Read the model definition and answer for the solid it produces. Units are mm, in the model's axes. Face numbers are marked on the shaded views. A direction names the side the tool comes from. Give positions to 0.01 mm unless a question says otherwise; leave off trailing zeros. Order: outer loops, then holes, each group sorted by start corner. A loop starts at its lowest first (then second) coordinate and runs counter-clockwise, first axis right, second up.
Item 1: A cutting plane is placed at D-D (z = 7). Write down the section's boundary in (x, y), plus the area to 3 significant figures.
Item 2: Find the intervals of material crossed by line 1 along X through (y, z) = (11, 24.5); line 2 along Z through (x, y) = (32.5, 3.5); line 3 along Y through (x, z) = (24, 1), in increasing order.
Item 3: Which of the six approach directions +Z, -Z, +X, -X, +Y, -Y give full straight-line access (tool end or side, diameter ignored) to the marked faces 1, 2 and 3?
Item 4: A cutting plane is placed at C-C (y = 10). Write down the section's boundary in (x, z).
Item 5: A cutting plane is placed at B-B (x = 19.5). Write down the section's boundary in (y, z).
Item 6: Given pin 1 Ø6 at (x, z) = (34.5, 20.5) entering from +Y; pin 2 Ø1 at (x, y) = (27, 40.5) entering from -Z; pin 3 Ø6 at (x, z) = (21, 26.5) entering from +Y; pin 4 Ø2 at (y, z) = (36.5, 33.5) entering from -X, each flat-ended and moving along its own axis, determine where each tip first touches the part or whether it passes through.
Item 7: The mould has two halves that part along Y. Classify the marked faces 4, 5, 6 and 7: +Y half, -Y half, draft (parallel to the pull), parting line (faces both ways), or undercut.
Item 8: A cutting plane is placed at A-A (z = 39.5). Write down the section's boundary in (x, y), plus the area to 3 significant figures.
from build123d import *

# Parameters (mm, degrees)
BOSS_EXTRUDE1_DEPTH      = 24.000000335
SKETCH2_W                = 24.000000671
SKETCH2_H                = 21.641136132
BOSS_EXTRUDE2_DEPTH      = 14.161821686
BOSS_EXTRUDE3_DEPTH      = 2.999999665
BOSS_EXTRUDE4_DEPTH      = 21.358863868
SKETCH5_W                = 27.000000671
SKETCH5_H                = 43
BOSS_EXTRUDE5_DEPTH      = 24.000001
CUT_EXTRUDE1_DEPTH       = 6.152247735
SKETCH7_W                = 24.000000671
SKETCH7_H                = 40
CUT_EXTRUDE2_DEPTH       = 8.00957395
BOSS_EXTRUDE6_START      = 3
BOSS_EXTRUDE6_DEPTH      = 3
SKETCH9_W                = 41
SKETCH9_H                = 22.000001
CUT_EXTRUDE3_DEPTH       = 66.345237915
SKETCH10_W               = 29.947000182
SKETCH10_H               = 17
BOSS_EXTRUDE7_DEPTH      = 2
F_5_0_5_DIAMETER_HOLE1_D = 5
FILLET1_R                = 1.5
FILLET2_R                = 5
SKETCH15_R               = 1.225
BOSS_EXTRUDE8_DEPTH      = 2


with BuildPart() as part:
    # Sketch1 → Boss-Extrude1 (new body)
    with BuildSketch(Plane(origin=(18, 0, 0), x_dir=(0, -1, 0), z_dir=(-1, 0, 0))):
        with BuildLine():
            Line((-0.838178314, 3), (-0.838178314, 0))
            Line((-0.838178314, 0), (0, 0))
            ThreePointArc((0, 0), (-0.41433113, 1.501329358), (-0.838178314, 3))
        make_face()
    extrude(amount=-BOSS_EXTRUDE1_DEPTH)

    # Sketch2 → Boss-Extrude2 (add)
    with BuildSketch(Plane(origin=(0, 0.838178314, 0), x_dir=(-1, 0, 0), z_dir=(0, 1, 0))):
        with Locations((-30.000000336, 10.820568066)):
            Rectangle(SKETCH2_W, SKETCH2_H)
    extrude(amount=BOSS_EXTRUDE2_DEPTH)


with BuildPart() as boss_extrude3_tool:
    # Sketch3 → Boss-Extrude3 (new body)
    with BuildSketch(Plane(origin=(42.000000335, 0, 0), x_dir=(0, 0, -1), z_dir=(1, 0, 0))):
        with BuildLine():
            Line((0, 15), (0, 0))
            ThreePointArc((0, 0), (-10.901557165, 3.244484944), (-21.641136132, 6.99042605))
            Line((-21.641136132, 6.99042605), (-43, 15))
            Line((-43, 15), (0, 15))
        make_face()
    extrude(amount=BOSS_EXTRUDE3_DEPTH)


with BuildPart() as part_1:
    add(part.part)


with BuildPart() as part_2:
    # Boss-Extrude3: joined with boss_extrude3_tool
    add(part_1.part.fuse(boss_extrude3_tool.part, tol=0.00001))

    # Sketch4 → Boss-Extrude4 (add)
    with BuildSketch(Plane.XY.offset(21.641136132)):
        Polygon((42.000000671, 15), (42.000000671, 6.99042605), (42.000000671, 0.838178314), (18, 0.838178314), (18, 6.99042605), (18, 15), align=None)
    extrude(amount=BOSS_EXTRUDE4_DEPTH)

    # Sketch5 → Boss-Extrude5 (add)
    with BuildSketch(Plane(origin=(0, 15, 0), x_dir=(-1, 0, 0), z_dir=(0, 1, 0))):
        with Locations((-31.500000336, 21.5)):
            Rectangle(SKETCH5_W, SKETCH5_H)
    extrude(amount=BOSS_EXTRUDE5_DEPTH)

    # Sketch6 → Cut-Extrude1 (cut)
    with BuildSketch(Plane.XZ.offset(-0.838178314)):
        Polygon((18, 3), (42.000000671, 3), (42.000000671, 21.641136132), (42.000000671, 43), (18, 43), align=None)
    extrude(amount=-CUT_EXTRUDE1_DEPTH, mode=Mode.SUBTRACT)

    # Sketch7 → Cut-Extrude2 (cut)
    with BuildSketch(Plane.XZ.offset(-6.99042605)):
        with Locations((30.000000336, 23)):
            Rectangle(SKETCH7_W, SKETCH7_H)
    extrude(amount=-CUT_EXTRUDE2_DEPTH, mode=Mode.SUBTRACT)

    # Sketch8 → Boss-Extrude6 (add)
    with BuildSketch(Plane.ZY.offset(-18).offset(BOSS_EXTRUDE6_START)):
        with BuildLine():
            Line((0, 39.000001), (43, 39.000001))
            Line((43, 39.000001), (43, 15))
            Line((43, 15), (21.641136132, 6.99042605))
            ThreePointArc((21.641136132, 6.99042605), (10.901557165, 3.244484944), (0, 0))
            Line((0, 0), (0, 39.000001))
        make_face()
    extrude(amount=-BOSS_EXTRUDE6_DEPTH)

    # Sketch9 → Cut-Extrude3 (cut, through all)
    with BuildSketch(Plane.ZY.offset(-15)):
        with Locations((20.5, 28.0000005)):
            Rectangle(SKETCH9_W, SKETCH9_H)
    extrude(amount=-CUT_EXTRUDE3_DEPTH, mode=Mode.SUBTRACT)

    # Sketch10 → Boss-Extrude7 (add)
    with BuildSketch(Plane(origin=(0, 39.000001, 0), x_dir=(-1, 0, 0), z_dir=(0, 1, 0))):
        with Locations((-30.02650058, 34.5)):
            Rectangle(SKETCH10_W, SKETCH10_H)
    extrude(amount=BOSS_EXTRUDE7_DEPTH)

    # 5.0 _5_ Diameter Hole1 (through all)
    with Locations(Plane.XY.offset(3)):
        with Locations((36.000000045, 10), (23.999999955, 10)):
            Hole(F_5_0_5_DIAMETER_HOLE1_D / 2)

    # Fillet1
    fillet1_edges = [part_2.edges().sort_by_distance(p)[0] for p in [
        (30.02650058, 41.000001, 43),
    ]]
    fillet(fillet1_edges, radius=FILLET1_R)

    # Fillet2
    fillet2_edges = [part_2.edges().sort_by_distance(p)[0] for p in [
        (30.02650058, 39.000001, 41),
        (30.000000335, 17, 41),
    ]]
    fillet(fillet2_edges, radius=FILLET2_R)

    # Sketch15 → Boss-Extrude8 (add)
    with BuildSketch(Plane(origin=(0, 41.000001, 0), x_dir=(1, 0, 0), z_dir=(0, 1, 0))):
        with Locations(Location((25.053000489, -39.5, 0), (0, 0, 90))):
            Circle(SKETCH15_R)
        with Locations(Location((35.053000489, -39.5, 0), (0, 0, 90))):
            Circle(SKETCH15_R)
    extrude(amount=BOSS_EXTRUDE8_DEPTH)


solid = part_2.part
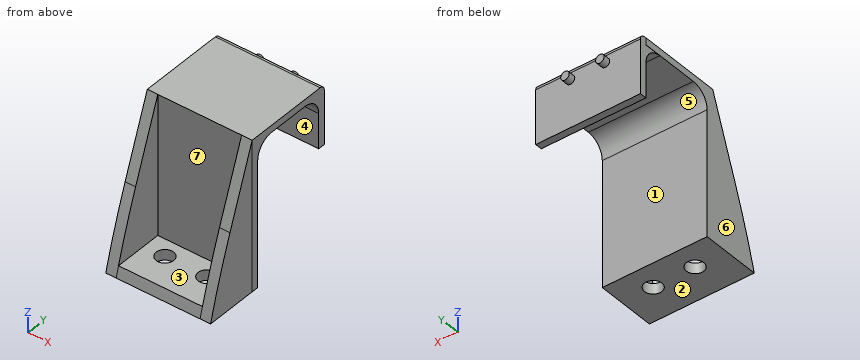
Response values:
1. outline: (15, 2.02) - (18, 2.02) - (18, 15) - (42, 15) - (42, 2.02) - (45, 2.02) - (45, 17) - (15, 17) - close
1. area: 138 mm2
2. line 1: x = 15 to 18, 42 to 45
2. line 2: z = 0 to 3
2. line 3: y = 0.27 to 7.5, 12.5 to 17
3. face 1: -Z, +X, -X
3. face 2: -Z, +X, -X, +Y, -Y
3. face 3: +Z, -Y
4. outline: (15, 0) - (21.5, 0) - (21.5, 3) - (18, 3) - (18, 29.67) - (15, 29.67) - close; (26.5, 0) - (33.5, 0) - (33.5, 3) - (26.5, 3) - close; (38.5, 0) - (45, 0) - (45, 29.67) - (42, 29.67) - (42, 3) - (38.5, 3) - close
5. outline: (0, 0) - (17, 0) - (17, 36) arc R5 cw to (22, 41) - (34, 41) arc R5 cw to (39, 36) - (39, 26) - (41, 26) - (41, 41.5) arc R1.5 ccw to (39.5, 43) - (15, 43) - (15, 3) - (0.84, 3) arc R245.5 ccw to start
6. pin 1: stops at y = 17
6. pin 2: stops at z = 26
6. pin 3: stops at y = 41
6. pin 4: passes through
7. face 4: undercut
7. face 5: undercut
7. face 6: draft
7. face 7: -Y half
8. outline: (15, 13.69) - (18, 13.69) - (18, 15) - (42, 15) - (42, 13.69) - (45, 13.69) - (45, 18.43) - (15, 18.43) - close; (15.05, 37.57) - (45, 37.57) - (45, 41) - (36.28, 41) - (36.28, 43) - (33.83, 43) - (33.83, 41) - (26.28, 41) - (26.28, 43) - (23.83, 43) - (23.83, 41) - (15.05, 41) - close
8. area: 223 mm2
